from build123d import *

# Parameters (mm, degrees)
EXTRUDE_1_DEPTH = 5
SKETCH_2_R      = 10
EXTRUDE_2_DEPTH = 46
SKETCH_4_W      = 35
SKETCH_4_H      = 30
EXTRUDE_3_DEPTH = 5
SKETCH_5_R      = 12.5
SKETCH_5_R_2    = 8
EXTRUDE_4_DEPTH = 200


with BuildPart() as part:
    # 草图1 → 凸台-拉伸1 (new body)
    with BuildSketch(Plane.XY):
        with BuildLine():
            Line((-17.5, 0), (-17.5, 40))
            Line((-17.5, 40), (17.5, 40))
            Line((17.5, 40), (17.5, 0))
            ThreePointArc((17.5, 0), (0, -17.5), (-17.5, 0))
        make_face()
    extrude(amount=EXTRUDE_1_DEPTH)

    # 草图2 → 凸台-拉伸2 (add)
    with BuildSketch(Plane.XY.offset(5)):
        Circle(SKETCH_2_R)
    extrude(amount=EXTRUDE_2_DEPTH)

    # 草图4 → 凸台-拉伸3 (add)
    with BuildSketch(Plane(origin=(0, 40, 0), x_dir=(1, 0, 0), z_dir=(0, 1, 0))):
        with Locations((0, -15)):
            Rectangle(SKETCH_4_W, SKETCH_4_H)
    extrude(amount=EXTRUDE_3_DEPTH)

    # 草图5 → 凸台-拉伸4 (add)
    with BuildSketch(Plane(origin=(0, 45, 0), x_dir=(1, 0, 0), z_dir=(0, 1, 0))):
        with Locations(Location((0, -15, 0), (0, 0, 270))):
            Circle(SKETCH_5_R)
        with Locations(Location((0, -15, 0), (0, 0, 270))):
            Circle(SKETCH_5_R_2, mode=Mode.SUBTRACT)
    extrude(amount=EXTRUDE_4_DEPTH)


solid = part.part
Could you check a few things on this model? Use its own coordinates, in mm. A direction names the side the tool comes from. Coordinates: 2 decimals unless noted, no trailing zeros. Order: outer loops, then holes, each group sorted by start corner. A loop starts at its lowest first (then second) coordinate and runs counter-clockwise, first axis right, second up. Notation, with made-up numbers: (-9, 56) -> (39, 56) arc R19 ccw to (39, 88) -> close; hole circle Ø2 at (26, -8.75). An arc over 180 degrees is marked (long way). One line per question, with ' | ' between items.
Q1. Imagine slicing it at A-A on z = 15. Please give me the cut outline in (x, y), and give its area (3 significant figures).
Return value:
outline: (-17.5, 40) -> (17.5, 40) -> (17.5, 45) -> (12.5, 45) -> (12.5, 245) -> (8, 245) -> (8, 45) -> (-8, 45) -> (-8, 245) -> (-12.5, 245) -> (-12.5, 45) -> (-17.5, 45) -> close; circle Ø20 at (0, 0) | area: 2,290 mm²
Q2. I'm going to push flat-ended pins straight in: P1, Ø8, axis at x = 3.5, z = 14.5, coming from the +Y side; P2, Ø2, axis at x = 9.5, y = 90.5, coming from the -Z side; P3, Ø20, axis at x = -7, z = 19, coming from the -Y side. Where does each tip first touch, or does it pass through?
Return value:
P1: y = 45 | P2: z = 5.83 | P3: y = -10
Q3. Imagine slicing it at D-D on x = 15. Please give me the cut outline in (y, z).
Return value:
outline: (-9.01, 0) -> (45, 0) -> (45, 30) -> (40, 30) -> (40, 5) -> (-9.01, 5) -> close
Q4. Imagine slicing it at B-B on y = 91.5. Please give me the cut outline in (x, z).
Return value:
outline: circle Ø25 at (0, 15); hole circle Ø16 at (0, 15)
Q5. On a 3-axis mill with a long thin cutter (end or side, diameter ignored), from which of +Z, -Z, +X, -X, +Y, -Y can I reach the whole of each face in a straight line? I mean faces 4 (the face through (0, 42, 30)), 5 (the face through (0, 40, 17)), 6 (the face through (-8, 45, 5)). Say none if no direction works.
Return value:
face 4: +Z, +X, -X, +Y | face 5: +Z, +X, -X | face 6: +Y
Q6. If I drill on L1, parallel to X at y = 171, z = 15; L2, parallel to Y at x = -1, z = 16; L3, parallel to Y at x = 1, z = 42, over which ranges is the centre line in solid material (lowest first)?
Return value:
L1: -12.5 to -8, 8 to 12.5 | L2: -9.95 to 9.95, 40 to 45 | L3: -9.95 to 9.95
Q7. Imagine slicing it at C-C on z = 44. Please give me the cut outline in (x, y), and give its area (3 significant figures).
Return value:
outline: circle Ø20 at (0, 0) | area: 314 mm²
Q8. Thinking about a two-plate mould opening in X: for faces 1 (the face through (-17.5, 31, 4)), 2 (the face through (8.45, 143.6, 5.79)), 3 (the face through (-4.868, 143.6, 8.651)), which applies, pulls with the +X half, pulls with the -X half, needs draft (parallel to the pull), parting line crosses it, or undercut?
Return value:
face 1: pulls with the -X half | face 2: parting line crosses it | face 3: undercut
